Here's how the part is built. I have some questions about the finished solid (model axes, mm). A direction names the side the tool comes from. Round coordinates to 2 decimals unless told otherwise and drop trailing zeros. Write each loop counter-clockwise with the first axis right and the second up, starting at its lowest first coordinate (ties: lowest second). Pieces come first, ordered by that corner, then holes. Notation, with made-up numbers: (-18, -10.75) - (-12, -10.75) arc R33 cw to (-12, 27.25) - close; hole circle Ø6 at (1.5, 32.5). An arc over 180 degrees is marked (long way). One line per question, with ' | ' between items. Start each with the question number.
(1) Imagine slicing it at A-A (x = 0.5). Write out the boundary of the cut face in (y, z) (3 decimals).
(2) Imagine slicing it at B-B (x = -65). Write out the boundary of the cut face in (y, z).
(3) Will these pins go through, and if not, where does the flat tip stop? pin 1 (6 mm diameter, centred on y = -5, z = -1, fed in from -X); pin 2 (7 mm diameter, centred on x = -9.5, z = 11, fed in from -Y); pin 3 (8 mm diameter, centred on x = -36.5, z = -6, fed in from +Y).
(4) For faces 1 (the flat face through (-41, -6, 7)), 2 (the cylindrical face through (-0.683, -2.958, 12.855)), which set-ups out of +Z, -Z, +X, -X, +Y, -Y let a thin tool reach every point of the face, with its end or its side?
(5) If I drill on L1, parallel to X at y = -1.75, z = -13; L2, parallel to Z at x = -42.5, y = -7.75 (3 decimals); L3, parallel to X at y = -2.75, z = -3, over which ranges is the centre line in solid material (lowest first)?
(6) Thinking about a two-plate mould opening in X: for faces 3 (the cylindrical face through (-46.62, -8.03, -10.82)), 4 (the cylindrical face through (-67.36, -1.757, 0.021)), 5 (the cylindrical face through (-30.773, -8.028, 6.49)), which applies, pulls with the +X half, pulls with the -X half, needs draft (parallel to the pull), parting line crosses it, or undercut?
from build123d import *

# Parameters (mm, degrees)
F0_W           = 155
F0_H           = 34
F1_DEPTH       = 10
F2_W           = 61
F2_H           = 4.5
F2_W_2         = 70
F2_W_3         = 155
F2_H_2         = 2.5
F3_DEPTH       = 2
F5_D           = 4.4
F5_CBORE_D     = 8.25
F5_CBORE_DEPTH = 4
F7_D           = 4.4
F7_CSINK_D     = 8.96
F7_CSINK_ANGLE = 90
F9_D           = 6.8
F9_DEPTH       = 20
F9_TIP         = 2.0429261047


with BuildPart() as f1:
    # F0 (on Front) → F1 (new body)
    with BuildSketch(Plane.XZ):
        Rectangle(F0_W, F0_H)
    extrude(amount=F1_DEPTH)

    # F2 (on face) → F3 (join)
    with BuildSketch(Plane(origin=(0, 0, 0), x_dir=(-1, 0, 0), z_dir=(0, 1, 0))):
        with Locations((47, 14.75)):
            Rectangle(F2_W, F2_H)
        with Locations((-42.5, 14.75)):
            Rectangle(F2_W_2, F2_H)
        with Locations((0, -15.75)):
            Rectangle(F2_W_3, F2_H_2)
    extrude(amount=F3_DEPTH)

    # F5 (through all)
    with Locations(Plane.XZ.offset(10)):
        with Locations((-42.5, 9), (-27.5, 9), (-9.5, 11), (0.5, 11), (-27.5, -11), (-42.5, -11)):
            CounterBoreHole(F5_D / 2, F5_CBORE_D / 2, F5_CBORE_DEPTH)

    # F7 (through all)
    with Locations(Plane(origin=(0, 0, 0), x_dir=(-1, 0, 0), z_dir=(0, 1, 0))):
        with Locations((-47.5, -1), (-15, -1), (17.5, -1)):
            CounterSinkHole(F7_D / 2, F7_CSINK_D / 2, counter_sink_angle=F7_CSINK_ANGLE)

    # F9
    with Locations(Plane(origin=(-77.5, 0, 0), x_dir=(0, -1, 0), z_dir=(-1, 0, 0))):
        with Locations((5, -1)):
            Hole(F9_D / 2, depth=F9_DEPTH)
            with Locations((0, 0, -(F9_DEPTH + F9_TIP / 2))):  # 118° drill point
                Cone(0, F9_D / 2, F9_TIP, mode=Mode.SUBTRACT)


solid = f1.part
Check sheet entries:
1) outline: (-10, -17) - (2, -17) - (2, -14.5) - (0, -14.5) - (0, 8.8) - (-6, 8.8) - (-6, 6.875) - (-10, 6.875) - close; (-10, 15.125) - (-6, 15.125) - (-6, 13.2) - (0, 13.2) - (0, 17) - (-10, 17) - close
2) outline: (-10, -17) - (2, -17) - (2, -14.5) - (0, -14.5) - (0, 12.5) - (2, 12.5) - (2, 17) - (-10, 17) - close; hole circle Ø6.8 at (-5, -1)
3) pin 1: x = -57.26 | pin 2: y = -6 | pin 3: y = 0
4) face 1: -Y | face 2: +Y, -Y
5) L1: -77.5 to -43.42, -41.58 to -28.42, -26.58 to 77.5 | L2: -17 to -15.125, -6.875 to 4.875, 13.125 to 17 | L3: -57.27 to -18.42, -16.58 to 14.08, 15.92 to 46.58, 48.42 to 77.5
6) face 3: undercut | face 4: needs draft | face 5: undercut
